Verification items for the finished model (mm, model axes). A direction names the side the tool comes from. Coordinates: 2 decimals unless noted, no trailing zeros. Write item = value, one per line. Start each with the question number.
1. Cross-section at A-A on y = -3. Give the number of separate pieces and of enclosed holes in the cut face, plus the area to 3 significant figures.
2. Go/stop test with a flat-tipped pin: P1, Ø2, axis at x = 17.5, z = 8.5, coming from the +Y side. Record where the tip stops, or that it passes through.
3. Release check for a two-part mould opening along Z. For faces 1 (the flat face through (15, -13, -14.877)), 2 (the flat face through (40.513, -13, 10)), 3 (the flat face through (2.118, -13, 18)) record: +Z half, -Z half, draft (parallel to the pull), parting line (faces both ways), or undercut.
4. Thickness scan on line 1 along Z through (x, y) = (11.5, -17.75); line 2 along Z through (x, y) = (10.5, -23.5); line 3 along Z through (x, y) = (2.5, -11.5). Record the ranges inside material, lowest first. Write a range as from..to.
5. Set-up check for faces 4 (the flat face through (15, -13, 35.923)), 5 (the flat face through (3.88, -12.52, 2.2)): record each of +Z, -Z, +X, -X, +Y, -Y from which the full face is reachable in a straight line by a thin tool's end or side.
from build123d import *

# Parameters (mm, degrees)
F0_W     = 50.8
F0_H     = 50.8
F1_DEPTH = 25.4


with BuildPart() as f1:
    # F0 (on Front) → F1 (new body)
    with BuildSketch(Plane.XZ):
        with Locations((15.1133043692, 10.5228427142)):
            Rectangle(F0_W, F0_H)
        Polygon((6.0826331481, -0.7500971721), (6.0826331481, -1.6127783157), (0.5940071434, 0.7979768292), (0.5940071434, 1.3572574011), (6.0826331481, 4.0933456892), (6.0826331481, 3.2434585456), (1.61569943, 1.1233099724), align=None, mode=Mode.SUBTRACT)
        with BuildLine():
            add(Edge.make_bspline(
                [(11.7595137243, 4.9185586899), (12.4339402963, 4.3620196894), (12.4339402963, 3.3915034029)],
                knots=[0, 0, 0, 1, 1, 1], degree=2))
            add(Edge.make_bspline(
                [(12.4339402963, 3.3915034029), (12.4339402963, 2.5909645451), (11.9852364388, 2.0828599732)],
                knots=[0, 0, 0, 1, 1, 1], degree=2))
            add(Edge.make_bspline(
                [(11.9852364388, 2.0828599732), (11.5365325813, 1.5747554013), (10.714061152, 1.4029502583)],
                knots=[0, 0, 0, 1, 1, 1], degree=2))
            Line((10.714061152, 1.4029502583), (10.714061152, 1.3572574011))
            add(Edge.make_bspline(
                [(10.714061152, 1.3572574011), (11.71930401, 1.2329728296), (12.2045621533, 0.7184712577)],
                knots=[0, 0, 0, 1, 1, 1], degree=2))
            add(Edge.make_bspline(
                [(12.2045621533, 0.7184712577), (12.6898202965, 0.2039696859), (12.6898202965, -0.6294680291)],
                knots=[0, 0, 0, 1, 1, 1], degree=2))
            add(Edge.make_bspline(
                [(12.6898202965, -0.6294680291), (12.6898202965, -1.8229654587), (11.8618657244, -2.4663208878)],
                knots=[0, 0, 0, 1, 1, 1], degree=2))
            add(Edge.make_bspline(
                [(11.8618657244, -2.4663208878), (11.0339111523, -3.109676317), (9.5095974367, -3.109676317)],
                knots=[0, 0, 0, 1, 1, 1], degree=2))
            add(Edge.make_bspline(
                [(9.5095974367, -3.109676317), (8.8461371504, -3.109676317), (8.2950812928, -3.0091520312)],
                knots=[0, 0, 0, 1, 1, 1], degree=2))
            add(Edge.make_bspline(
                [(8.2950812928, -3.0091520312), (7.7440254352, -2.9086277454), (7.2249545776, -2.658230888)],
                knots=[0, 0, 0, 1, 1, 1], degree=2))
            Line((7.2249545776, -2.658230888), (7.2249545776, -1.7553400301))
            add(Edge.make_bspline(
                [(7.2249545776, -1.7553400301), (7.7677857209, -2.0240140303), (8.3818977214, -2.1638341733)],
                knots=[0, 0, 0, 1, 1, 1], degree=2))
            add(Edge.make_bspline(
                [(8.3818977214, -2.1638341733), (8.996009722, -2.3036543163), (9.5443240081, -2.3036543163)],
                knots=[0, 0, 0, 1, 1, 1], degree=2))
            add(Edge.make_bspline(
                [(9.5443240081, -2.3036543163), (11.7083377243, -2.3036543163), (11.7083377243, -0.6075354577)],
                knots=[0, 0, 0, 1, 1, 1], degree=2))
            add(Edge.make_bspline(
                [(11.7083377243, -0.6075354577), (11.7083377243, 0.9131228293), (9.3213428651, 0.9131228293)],
                knots=[0, 0, 0, 1, 1, 1], degree=2))
            Line((9.3213428651, 0.9131228293), (8.4988714358, 0.9131228293))
            Line((8.4988714358, 0.9131228293), (8.4988714358, 1.7282834015))
            Line((8.4988714358, 1.7282834015), (9.3323091508, 1.7282834015))
            add(Edge.make_bspline(
                [(9.3323091508, 1.7282834015), (10.3083085802, 1.7282834015), (10.879469295, 2.1596239733)],
                knots=[0, 0, 0, 1, 1, 1], degree=2))
            add(Edge.make_bspline(
                [(10.879469295, 2.1596239733), (11.4506300098, 2.5909645451), (11.4506300098, 3.3567768314)],
                knots=[0, 0, 0, 1, 1, 1], degree=2))
            add(Edge.make_bspline(
                [(11.4506300098, 3.3567768314), (11.4506300098, 3.9672334034), (11.0311695808, 4.3163268322)],
                knots=[0, 0, 0, 1, 1, 1], degree=2))
            add(Edge.make_bspline(
                [(11.0311695808, 4.3163268322), (10.6117091519, 4.6654202611), (9.8915897227, 4.6654202611)],
                knots=[0, 0, 0, 1, 1, 1], degree=2))
            add(Edge.make_bspline(
                [(9.8915897227, 4.6654202611), (9.3432754365, 4.6654202611), (8.8580172933, 4.5164615467)],
                knots=[0, 0, 0, 1, 1, 1], degree=2))
            add(Edge.make_bspline(
                [(8.8580172933, 4.5164615467), (8.37275915, 4.3675028323), (7.749508578, 3.9672334034)],
                knots=[0, 0, 0, 1, 1, 1], degree=2))
            Line((7.749508578, 3.9672334034), (7.2706474348, 4.6069334039))
            add(Edge.make_bspline(
                [(7.2706474348, 4.6069334039), (7.7842351495, 5.0126859757), (8.4550062929, 5.243891833)],
                knots=[0, 0, 0, 1, 1, 1], degree=2))
            add(Edge.make_bspline(
                [(8.4550062929, 5.243891833), (9.1257774364, 5.4750976904), (9.8696571513, 5.4750976904)],
                knots=[0, 0, 0, 1, 1, 1], degree=2))
            add(Edge.make_bspline(
                [(9.8696571513, 5.4750976904), (11.0850871523, 5.4750976904), (11.7595137243, 4.9185586899)],
                knots=[0, 0, 0, 1, 1, 1], degree=2))
        make_face(mode=Mode.SUBTRACT)
        Polygon((5.8029928621, 12.9138948396), (1.1478045724, 12.9138948396), (1.1478045724, 21.2647214181), (2.118320859, 21.2647214181), (2.118320859, 13.7930254118), (5.8029928621, 13.7930254118), align=None, mode=Mode.SUBTRACT)
        with BuildLine():
            add(Edge.make_bspline(
                [(13.4574602972, 20.2539954173), (14.4681862981, 19.1116739877), (14.4681862981, 17.1011882717)],
                knots=[0, 0, 0, 1, 1, 1], degree=2))
            add(Edge.make_bspline(
                [(14.4681862981, 17.1011882717), (14.4681862981, 15.0961856986), (13.4538048686, 13.947467269)],
                knots=[0, 0, 0, 1, 1, 1], degree=2))
            add(Edge.make_bspline(
                [(13.4538048686, 13.947467269), (12.4394234392, 12.7987488395), (10.6354694377, 12.7987488395)],
                knots=[0, 0, 0, 1, 1, 1], degree=2))
            add(Edge.make_bspline(
                [(10.6354694377, 12.7987488395), (8.7913057218, 12.7987488395), (7.7888044352, 13.9273624119)],
                knots=[0, 0, 0, 1, 1, 1], degree=2))
            add(Edge.make_bspline(
                [(7.7888044352, 13.9273624119), (6.7863031487, 15.0559759843), (6.7863031487, 17.1121545575)],
                knots=[0, 0, 0, 1, 1, 1], degree=2))
            add(Edge.make_bspline(
                [(6.7863031487, 17.1121545575), (6.7863031487, 19.1518837021), (7.7915460067, 20.2741002744)],
                knots=[0, 0, 0, 1, 1, 1], degree=2))
            add(Edge.make_bspline(
                [(7.7915460067, 20.2741002744), (8.7967888647, 21.3963168468), (10.6464357234, 21.3963168468)],
                knots=[0, 0, 0, 1, 1, 1], degree=2))
            add(Edge.make_bspline(
                [(10.6464357234, 21.3963168468), (12.4467342963, 21.3963168468), (13.4574602972, 20.2539954173)],
                knots=[0, 0, 0, 1, 1, 1], degree=2))
        make_face(mode=Mode.SUBTRACT)
        with BuildLine():
            Line((19.1910000164, 15.8948968421), (21.0991337323, 21.2647214181))
            Line((21.0991337323, 21.2647214181), (22.1427585903, 21.2647214181))
            Line((22.1427585903, 21.2647214181), (19.1343408735, 12.9138948396))
            Line((19.1343408735, 12.9138948396), (18.1747908727, 12.9138948396))
            Line((18.1747908727, 12.9138948396), (15.1809948701, 21.2647214181))
            Line((15.1809948701, 21.2647214181), (16.2099980138, 21.2647214181))
            Line((16.2099980138, 21.2647214181), (18.1290980155, 15.861997985))
            add(Edge.make_bspline(
                [(18.1290980155, 15.861997985), (18.4599143015, 14.9298636984), (18.6536520159, 14.0507331263)],
                knots=[0, 0, 0, 1, 1, 1], degree=2))
            add(Edge.make_bspline(
                [(18.6536520159, 14.0507331263), (18.8601837304, 14.9755565556), (19.1910000164, 15.8948968421)],
                knots=[0, 0, 0, 1, 1, 1], degree=2))
        make_face(mode=Mode.SUBTRACT)
        Polygon((27.9457514524, 13.782059126), (27.9457514524, 12.9138948396), (23.2905631627, 12.9138948396), (23.2905631627, 21.2647214181), (27.9457514524, 21.2647214181), (27.9457514524, 20.4020402746), (24.2610794493, 20.4020402746), (24.2610794493, 17.7116448437), (27.7227703094, 17.7116448437), (27.7227703094, 16.8544468429), (24.2610794493, 16.8544468429), (24.2610794493, 13.782059126), align=None, mode=Mode.SUBTRACT)
    extrude(amount=F1_DEPTH)


solid = f1.part
Worked out:
q1.separate_pieces = 1
q1.enclosed_holes = 6
q1.area = 2,460 mm²
q2.P1 = 0
q3.face_1 = -Z half
q3.face_2 = draft
q3.face_3 = undercut
q4.line_1 = -14.88..-2.7, -1.5..0.16, 1.17..1.69, 5.1..12.87, 21.32..35.92
q4.line_2 = -14.88..-3.03, -2.2..0.79, 1.94..4.59, 5.43..12.8, 21.39..35.92
q4.line_3 = -14.88..-0.04, 0.75..1.54, 2.31..12.91, 13.79..35.92
q5.face_4 = +Z, +X, -X, +Y, -Y
q5.face_5 = +Y, -Y
